Geometry: see drawing. Coordinates: mm, zero at the bounding-box minimum. A direction names the side the tool comes from. Round coordinates to 2 decimals unless told otherwise and drop trailing zeros. Order: outer loops, then holes, each group sorted by start corner. A loop starts at its lowest first (then second) coordinate and runs counter-clockwise, first axis right, second up. Notation, with made-up numbers: (86.25, -2) -> (103.25, -2) arc R36 cw to (103.25, 36) -> close; hole circle Ø8 at (46.5, 24). An arc over 180 degrees is marked (long way). Put each result on its own line as item: value.
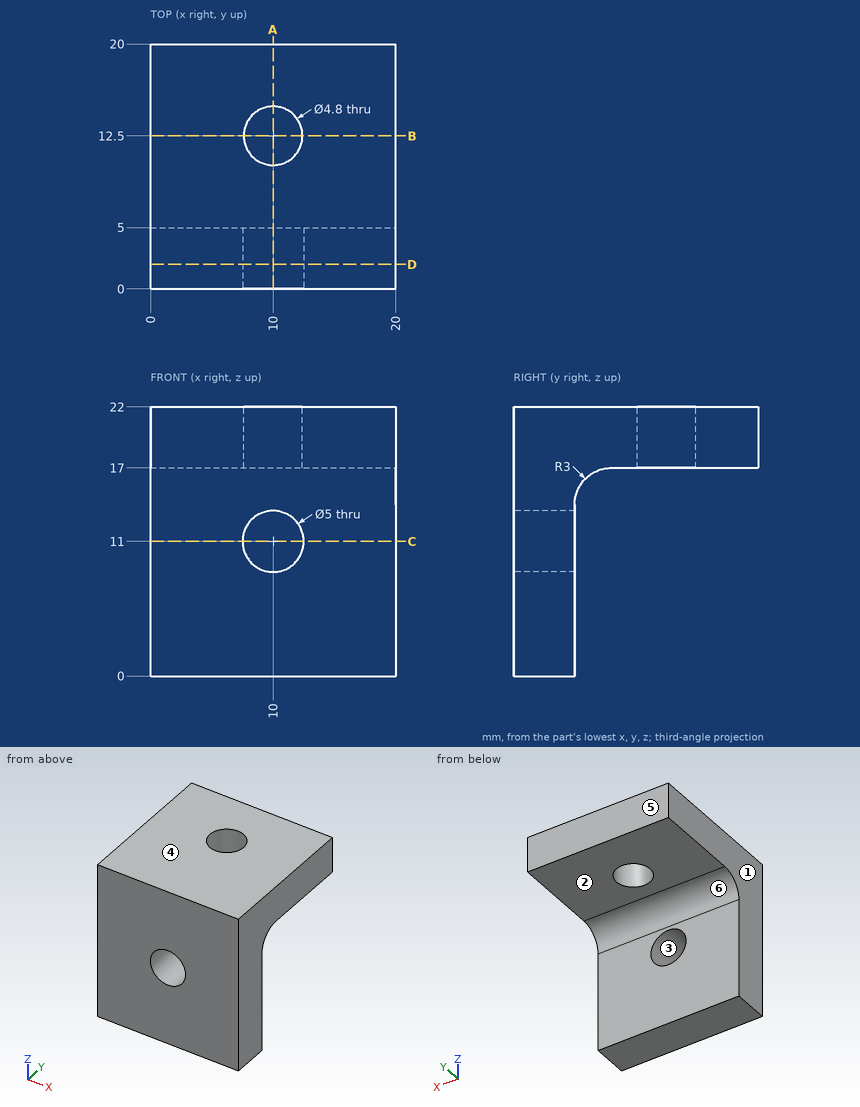
1. Material intervals for probe 1 along X at (y, z) = (2.2, 11); probe 2 along X at (y, z) = (12.5, 18.05); probe 3 along Y at (x, z) = (10, 18.6), sorted ascending.
Ans:
probe 1: 0 to 7.5, 12.5 to 20
probe 2: 0 to 7.6, 12.4 to 20
probe 3: 0 to 10.1, 14.9 to 20
2. Set-up query: the marked faces 1 and 2. Return all of +Z, -Z, +X, -X, +Y, -Y with unobstructed straight access to the full face (end or side cutting, diameter ignored); none if empty.
Ans:
face 1: +Z, -Z, -X, +Y, -Y
face 2: -Z, +X, -X, +Y
3. Cut plane A-A on x = 10. Return loops of the section in (y, z).
Ans:
outline: (0, 0) -> (5, 0) -> (5, 8.5) -> (0, 8.5) -> close; (0, 13.5) -> (5, 13.5) -> (5, 14) arc R3 cw to (8, 17) -> (10.1, 17) -> (10.1, 22) -> (0, 22) -> close; (14.9, 17) -> (20, 17) -> (20, 22) -> (14.9, 22) -> close
4. Cut plane D-D on y = 2. Return loops of the section in (x, z).
Ans:
outline: (0, 0) -> (20, 0) -> (20, 22) -> (0, 22) -> close; hole circle Ø5 at (10, 11)
5. Contact query for flat-ended pins moving along their axis: P1, Ø8, axis at x = 10.5, z = 6, coming from the +Y side; P2, Ø3.5, axis at x = 13.5, y = 12, coming from the -Z side. Output: stop coordinate, or through.
Ans:
P1: y = 5
P2: z = 17
6. Draft query along Z for the marked faces 3, 4, 5 and 6. Return one class per face: +Z half, -Z half, draft (parallel to the pull), parting line (faces both ways), or undercut.
Ans:
face 3: undercut
face 4: +Z half
face 5: draft
face 6: -Z half
7. Cut plane B-B on y = 12.5. Return loops of the section in (x, z).
Ans:
outline: (0, 17) -> (7.6, 17) -> (7.6, 22) -> (0, 22) -> close; (12.4, 17) -> (20, 17) -> (20, 22) -> (12.4, 22) -> close
8. Cut plane C-C on z = 11. Return loops of the section in (x, y).
Ans:
outline: (0, 0) -> (7.5, 0) -> (7.5, 5) -> (0, 5) -> close; (12.5, 0) -> (20, 0) -> (20, 5) -> (12.5, 5) -> close
